Geometry: see drawing. Coordinates: mm, zero at the bounding-box minimum. Give positions to 0.01 mm unless a question says otherwise; leave off trailing zeros. Order: outer loops, then holes, each group sorted by start corner. A loop starts at its lowest first (then second) coordinate and runs counter-clockwise, first axis right, second up. Notation, with made-up numbers: (75.5, -11) - (87.5, -11) arc R28 ccw to (87.5, 15) - close; hole circle Ø10 at (52, 60.25). An arc over 180 degrees is marked (long way). Write each question's results on one line, items separated by ' | '. Start each with the question number.
Item 1: Line query: line 1 along Y through (x, z) = (5, 10); line 2 along Z through (x, y) = (4, 3); line 3 along Y through (x, z) = (4.75, 3.5). Output: solid intervals per line, ascending.
Item 2: Section D-D on x = 2.75. Output: boundary loops of the cut face in (y, z), and give its area (3 significant figures).
Item 3: Contact query for flat-ended pins moving along their axis: pin 1 Ø5.5 at (x, y) = (4.5, 5.5) entering from +Z; pin 2 Ø4 at (x, z) = (1, 6) entering from +Y; pin 3 Ø4 at (y, z) = (8, 4.5) entering from +X; pin 4 Ø2 at (x, z) = (6, 8) entering from -Y. Output: stop coordinate, or through.
Item 4: Section A-A on x = 5. Output: boundary loops of the cut face in (y, z), and give its area (3 significant figures).
Item 5: Section C-C on z = 2.5. Output: boundary loops of the cut face in (x, y).
Item 6: Mould query, pull axis Y, two halves, no side actions, for the marked faces 1, 2 and 3. Classes: released by +Y, released by -Y, zero draft, split by the parting line, or undercut.
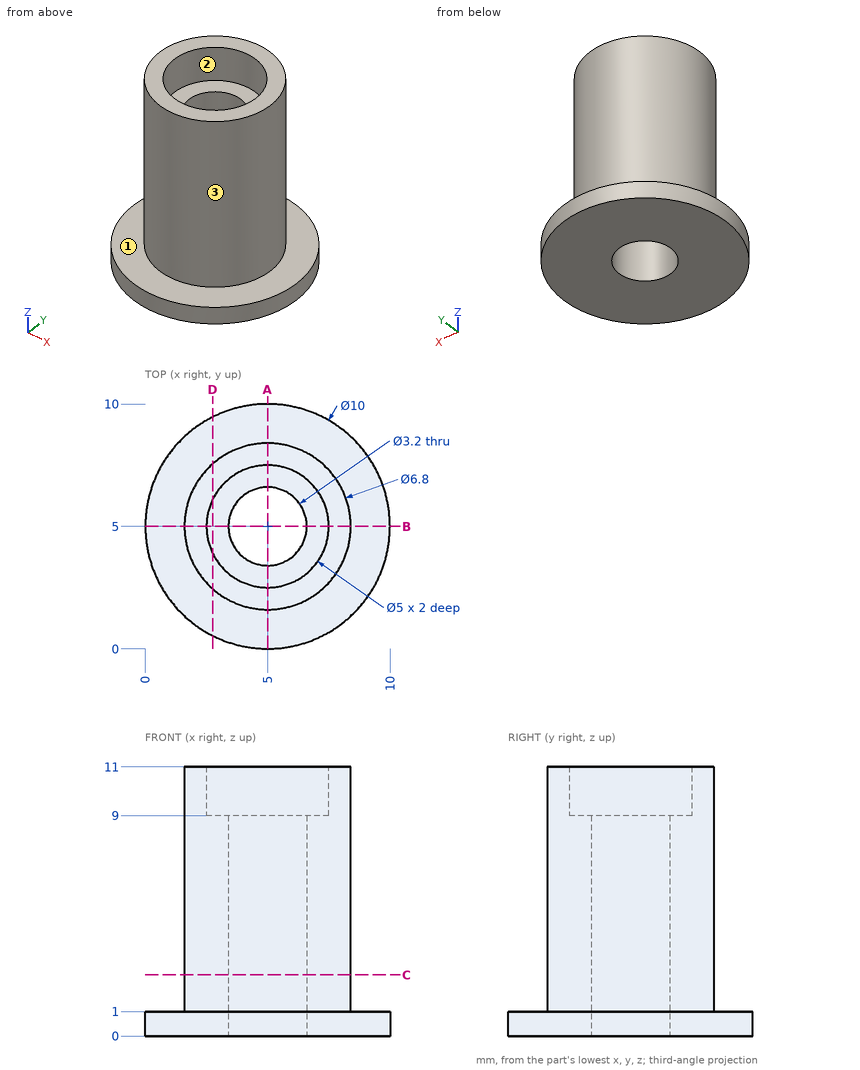
Evaluation:
1) line 1: y = 1.6 to 2.5, 7.5 to 8.4 | line 2: z = 0 to 9 | line 3: y = 1.61 to 3.42, 6.58 to 8.39
2) outline: (0.53, 0) - (9.47, 0) - (9.47, 1) - (7.55, 1) - (7.55, 11) - (6.09, 11) - (6.09, 9) - (3.91, 9) - (3.91, 11) - (2.45, 11) - (2.45, 1) - (0.53, 1) - close | area: 55.6 mm^2
3) pin 1: stops at z = 11 | pin 2: stops at y = 7.75 | pin 3: stops at x = 8.25 | pin 4: stops at y = 1.6
4) outline: (0, 0) - (3.4, 0) - (3.4, 9) - (2.5, 9) - (2.5, 11) - (1.6, 11) - (1.6, 1) - (0, 1) - close; (6.6, 0) - (10, 0) - (10, 1) - (8.4, 1) - (8.4, 11) - (7.5, 11) - (7.5, 9) - (6.6, 9) - close | area: 39.2 mm^2
5) outline: circle Ø6.8 at (5, 5); hole circle Ø3.2 at (5, 5)
6) face 1: zero draft | face 2: undercut | face 3: split by the parting line
